Model file for the job. Use its own axes, mm. Face numbers are marked on the shaded views. A direction names the side the tool comes from. Give positions to 0.01 mm unless a question says otherwise; leave off trailing zeros. Loops run counter-clockwise (first coordinate to the right, second up) from the corner with the lowest first, then second, coordinate; pieces in that order, holes last. Notation, with made-up numbers: (3, -19) - (28, -19) arc R33 cw to (28, 9) - close; hole circle Ø7 at (-28.5, 57.5). An arc over 180 degrees is marked (long way). Use a Markdown table: item, result.
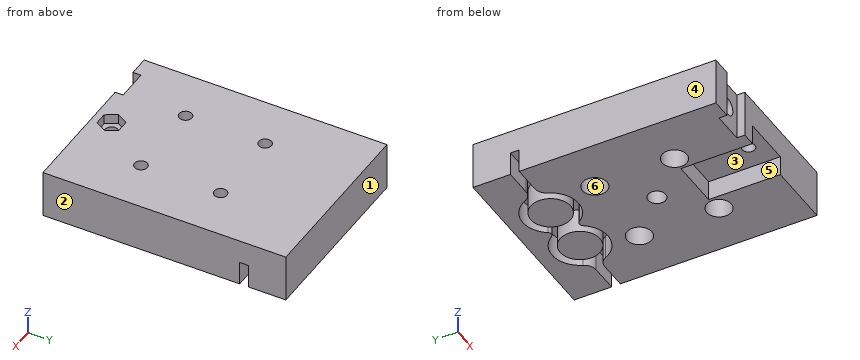
from build123d import *

# Parameters (mm, degrees)
SKETCH_1_W          = 45.4
SKETCH_1_H          = 27
EXTRUDE_1_DEPTH     = 7
SKETCH_2_R          = 1.6
CUT_EXTRUDE_1_DEPTH = 62.727033531
SKETCH_4_R          = 3.1
EXTRUDE_2_DEPTH     = 5
SKETCH_5_W          = 45.4
SKETCH_5_H          = 12
EXTRUDE_3_DEPTH     = 20
SKETCH_7_R          = 5
CUT_EXTRUDE_3_DEPTH = 6
EXTRUDE_4_DEPTH     = 14
SKETCH_9_R          = 1.6
CUT_EXTRUDE_4_DEPTH = 74.531810641
CUT_EXTRUDE_5_DEPTH = 2.5
SKETCH_10_W         = 8
SKETCH_10_H         = 12
CUT_EXTRUDE_6_DEPTH = 2
SKETCH_12_R         = 2.2
CUT_EXTRUDE_8_DEPTH = 6
SKETCH_13_R         = 2.2
CUT_EXTRUDE_9_DEPTH = 6


with BuildPart() as part:
    # 草图1 → 凸台-拉伸1 (new body)
    with BuildSketch(Plane.XY):
        with Locations((-32.096319797, 14.04251269)):
            Rectangle(SKETCH_1_W, SKETCH_1_H)
    extrude(amount=EXTRUDE_1_DEPTH)

    # 草图2 → 切除-拉伸1 (cut, through all)
    with BuildSketch(Plane(origin=(0, 0, 0), x_dir=(-1, 0, 0), z_dir=(0, 0, -1))):
        with Locations((22.096319797, 24.04251269)):
            Circle(SKETCH_2_R)
        with Locations(Location((42.096319797, 24.04251269, 0), (0, 0, 180))):
            Circle(SKETCH_2_R)
        with Locations((42.096319797, 4.04251269)):
            Circle(SKETCH_2_R)
        with Locations(Location((22.096319797, 4.04251269, 0), (0, 0, 180))):
            Circle(SKETCH_2_R)
    extrude(amount=-CUT_EXTRUDE_1_DEPTH, mode=Mode.SUBTRACT)

    # 草图4 → 凸台-拉伸2 (add)
    with BuildSketch(Plane(origin=(0, 0, 0), x_dir=(-1, 0, 0), z_dir=(0, 0, -1))):
        Polygon((38.346319797, 0.54251269), (54.796319797, 0.54251269), (54.796319797, 27.54251269), (9.396319797, 27.54251269), (9.396319797, 0.54251269), (25.846319797, 0.54251269), (25.846319797, 4.54251269), (38.346319797, 4.54251269), align=None)
        with Locations(Location((42.096319797, 24.04251269, 0), (0, 0, 180))):
            Circle(SKETCH_4_R, mode=Mode.SUBTRACT)
        with Locations((22.096319797, 24.04251269)):
            Circle(SKETCH_4_R, mode=Mode.SUBTRACT)
        with Locations((42.096319797, 4.04251269)):
            Circle(SKETCH_4_R, mode=Mode.SUBTRACT)
        with Locations(Location((22.096319797, 4.04251269, 0), (0, 0, 180))):
            Circle(SKETCH_4_R, mode=Mode.SUBTRACT)
    extrude(amount=EXTRUDE_2_DEPTH)

    # 草图5 → 凸台-拉伸3 (add)
    with BuildSketch(Plane(origin=(0, 27.54251269, 0), x_dir=(1, 0, 0), z_dir=(0, 1, 0))):
        with Locations((-32.096319797, -1)):
            Rectangle(SKETCH_5_W, SKETCH_5_H)
    extrude(amount=EXTRUDE_3_DEPTH)

    # 草图7 → 切除-拉伸3 (cut)
    with BuildSketch(Plane(origin=(0, 0, -5), x_dir=(-1, 0, 0), z_dir=(0, 0, -1))):
        with BuildLine():
            Line((9.396319797, 38.14251269), (16.375464574, 38.14251269))
            ThreePointArc((16.375464574, 38.14251269), (18.004881648, 38.623584347), (19.111721141, 39.91251269))
            ThreePointArc((19.111721141, 39.91251269), (24.873653651, 44.014763896), (31.271319797, 40.998441785))
            ThreePointArc((31.271319797, 40.998441785), (32.096319797, 40.563574513), (32.921319797, 40.998441785))
            ThreePointArc((32.921319797, 40.998441785), (39.318985943, 44.014763896), (45.080918453, 39.91251269))
            ThreePointArc((45.080918453, 39.91251269), (46.187757946, 38.623584347), (47.81717502, 38.14251269))
            Line((47.81717502, 38.14251269), (54.796319797, 38.14251269))
            Line((54.796319797, 38.14251269), (54.796319797, 35.94251269))
            Line((54.796319797, 35.94251269), (47.81717502, 35.94251269))
            ThreePointArc((47.81717502, 35.94251269), (46.187757946, 35.461441034), (45.080918453, 34.17251269))
            ThreePointArc((45.080918453, 34.17251269), (39.318985943, 30.070261485), (32.921319797, 33.086583596))
            ThreePointArc((32.921319797, 33.086583596), (32.096319797, 33.521450868), (31.271319797, 33.086583596))
            ThreePointArc((31.271319797, 33.086583596), (24.873653651, 30.070261485), (19.111721141, 34.17251269))
            ThreePointArc((19.111721141, 34.17251269), (18.004881648, 35.461441034), (16.375464574, 35.94251269))
            Line((16.375464574, 35.94251269), (9.396319797, 35.94251269))
            Line((9.396319797, 35.94251269), (9.396319797, 38.14251269))
        make_face()
        with Locations((25.496319797, 37.04251269)):
            Circle(SKETCH_7_R, mode=Mode.SUBTRACT)
        with Locations(Location((38.696319797, 37.04251269, 0), (0, 0, 180))):
            Circle(SKETCH_7_R, mode=Mode.SUBTRACT)
    extrude(amount=-CUT_EXTRUDE_3_DEPTH, mode=Mode.SUBTRACT)

    # 草图8 → 凸台-拉伸4 (add)
    with BuildSketch(Plane.XZ.offset(-0.54251269)):
        Polygon((-38.346319797, -5), (-38.346319797, 0), (-25.846319797, 0), (-25.846319797, -5), (-9.396319797, -5), (-9.396319797, 7), (-54.796319797, 7), (-54.796319797, -5), align=None)
    extrude(amount=EXTRUDE_4_DEPTH)

    # 草图9 → 切除-拉伸4 (cut, through all)
    with BuildSketch(Plane.XY.offset(7)):
        with Locations((-32.096319797, -8.95748731)):
            Circle(SKETCH_9_R)
    extrude(amount=-CUT_EXTRUDE_4_DEPTH, mode=Mode.SUBTRACT)

    # 草图3 → 切除-拉伸5 (cut)
    with BuildSketch(Plane.XY.offset(7)):
        Polygon((-28.920893316, -8.95748731), (-30.508606557, -6.20748731), (-33.684033037, -6.20748731), (-35.271746277, -8.95748731), (-33.684033037, -11.70748731), (-30.508606557, -11.70748731), align=None)
    extrude(amount=-CUT_EXTRUDE_5_DEPTH, mode=Mode.SUBTRACT)

    # 草图10 → 切除-拉伸6 (cut)
    with BuildSketch(Plane.XZ.offset(13.45748731)):
        with Locations((-45.796319797, 1)):
            Rectangle(SKETCH_10_W, SKETCH_10_H)
    extrude(amount=-CUT_EXTRUDE_6_DEPTH, mode=Mode.SUBTRACT)

    # 草图12 → 切除-拉伸8 (cut)
    with BuildSketch(Plane.XZ.offset(11.45748731)):
        with Locations(Location((-45.796319797, 1, 0), (0, 0, 270))):
            Circle(SKETCH_12_R)
    extrude(amount=-CUT_EXTRUDE_8_DEPTH, mode=Mode.SUBTRACT)

    # 草图13 → 切除-拉伸9 (cut)
    with BuildSketch(Plane(origin=(0, 0, -5), x_dir=(-1, 0, 0), z_dir=(0, 0, -1))):
        with Locations((32.096319797, 14.04251269)):
            Circle(SKETCH_13_R)
    extrude(amount=-CUT_EXTRUDE_9_DEPTH, mode=Mode.SUBTRACT)


solid = part.part
(1) 3-axis set-ups, long thin cutter, end or side, ignore diameter. For the marked faces 4, 5 and 6: which of +Z, -Z, +X, -X, +Y, -Y reach the whole face in a straight line?
Computed:
| item | result |
|---|---|
| face 4 | +Z, -Z, -X, +Y, -Y |
| face 5 | -Z, -Y |
| face 6 | -Z |
(2) Slice it at C-C, the plane x = -23. Write the cut outline in (y, z), plus the area to 3 significant figures.
Computed:
| item | result |
|---|---|
| outline | (-13.46, -5) - (1.08, -5) - (1.08, 0) - (2.72, 0) - (2.72, 7) - (-13.46, 7) - close; (5.36, 0) - (7.01, 0) - (7.01, -5) - (21.08, -5) - (21.08, 0) - (22.72, 0) - (22.72, 7) - (5.36, 7) - close; (25.36, 0) - (27.01, 0) - (27.01, -5) - (30.5, -5) - (30.5, 1) - (32.71, 1) - (32.71, -5) - (41.37, -5) - (41.37, 1) - (43.58, 1) - (43.58, -5) - (47.54, -5) - (47.54, 7) - (25.36, 7) - close |
| area | 609 mm² |
(3) Slice it at A-A, the plane x = -52. Write the cut outline in (y, z).
Computed:
| item | result |
|---|---|
| outline | (-13.46, -5) - (35.94, -5) - (35.94, 1) - (38.14, 1) - (38.14, -5) - (47.54, -5) - (47.54, 7) - (-13.46, 7) - close |
(4) Slice it at B-B, the plane z = 5.5. Write the cut outline in (x, y), plus the area to 3 significant figures.
Computed:
| item | result |
|---|---|
| outline | (-54.8, -13.46) - (-49.8, -13.46) - (-49.8, -11.46) - (-41.8, -11.46) - (-41.8, -13.46) - (-9.4, -13.46) - (-9.4, 47.54) - (-54.8, 47.54) - close; hole circle Ø3.2 at (-42.1, 4.04); hole circle Ø3.2 at (-42.1, 24.04); hole (-35.27, -8.96) - (-33.68, -11.71) - (-30.51, -11.71) - (-28.92, -8.96) - (-30.51, -6.21) - (-33.68, -6.21) - close; hole circle Ø3.2 at (-22.1, 4.04); hole circle Ø3.2 at (-22.1, 24.04) |
| area | 2,700 mm² |
(5) Pin check, flat tips, straight feed: P1, Ø5, axis at x = -32.1, y = -8.96, coming from the -Z side; P2, Ø3.5, axis at x = -46, z = 1.5, coming from the -Y side; P3, Ø1.3, axis at x = -31, y = 13.5, coming from the -Z side. Stop position of each tip, or through.
Computed:
| item | result |
|---|---|
| P1 | z = 0 |
| P2 | y = -11.46 |
| P3 | z = 1 |
(6) Slice it at D-D, the plane y = -4.5. Write the cut outline in (x, z), plus the area to 3 significant figures.
Computed:
| item | result |
|---|---|
| outline | (-54.8, -5) - (-38.35, -5) - (-38.35, 0) - (-25.85, 0) - (-25.85, -5) - (-9.4, -5) - (-9.4, 7) - (-54.8, 7) - close |
| area | 482 mm² |
(7) Mould opens along X. For the marked faces 1, 2 and 3 say: pulls with the +X half, pulls with the -X half, needs draft (parallel to the pull), parting line crosses it, or undercut.
Computed:
| item | result |
|---|---|
| face 1 | needs draft |
| face 2 | pulls with the +X half |
| face 3 | undercut |
(8) Drill centre lines: probe 1 along X at (y, z) = (-6.95, 1); probe 2 along X at (y, z) = (-8.05, 1); probe 3 along X at (y, z) = (-8.5, 1.25). Where is each one in solid material? Low to high. Write a range as [from, to].
Computed:
| item | result |
|---|---|
| probe 1 | [-54.8, -48], [-43.6, -9.4] |
| probe 2 | [-54.8, -48], [-43.6, -33.41], [-30.78, -9.4] |
| probe 3 | [-54.8, -47.98], [-43.61, -33.63], [-30.56, -9.4] |
